Verification items for the finished model (mm, model axes). Face numbers are marked on the shaded views. A direction names the side the tool comes from. Give positions to 0.01 mm unless a question says otherwise; leave off trailing zeros. Loops run counter-clockwise (first coordinate to the right, second up) from the corner with the lowest first, then second, coordinate; pieces in that order, holes last. Notation, with made-up numbers: M -14.75,39.25 L 8.25,39.25 A19 cw 8.25,54.25 Z; hole C -0.5,73.25 d3. An arc over 180 degrees is marked long. Use CSV: the item, a comma, the result in double quotes.
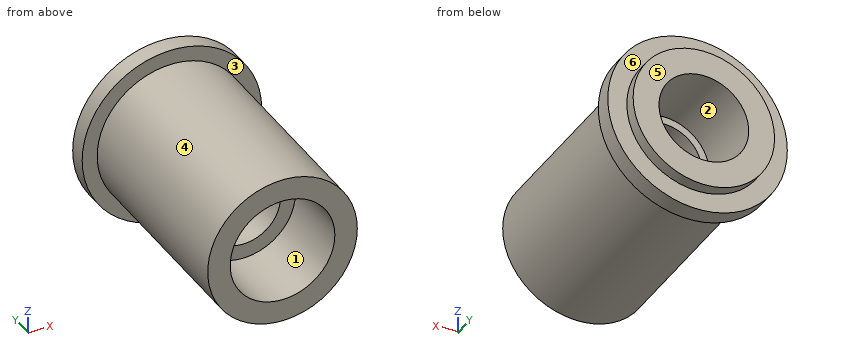
from build123d import *

# Parameters (mm, degrees)
F0_R     = 9.525
F0_R_2   = 7.5057
F0_R_3   = 4.7625
F1_DEPTH = 25.4
F2_R     = 5.55625
F3_DEPTH = 7.9375
F2_R_2   = 9.525
F2_R_3   = 7.9375
F5_DEPTH = 22.225
F6_DEPTH = 1.27
F7_DEPTH = 7.9375
F8_D     = 7.9375


with BuildPart() as f1:
    # F0 (on Front) → F1 (new body)
    with BuildSketch(Plane.XZ):
        Circle(F0_R)
        Circle(F0_R_2, mode=Mode.SUBTRACT)
        Circle(F0_R_2)
        Circle(F0_R_3, mode=Mode.SUBTRACT)
        Circle(F0_R_3)
    extrude(amount=F1_DEPTH)

    # F2 (on face) → F3 (cut)
    with BuildSketch(Plane.XZ.offset(25.4)):
        Circle(F2_R)
    extrude(amount=-F3_DEPTH, mode=Mode.SUBTRACT)

    # F2 (on face) → F5 (cut)
    with BuildSketch(Plane.XZ.offset(25.4)):
        Circle(F2_R_2)
        Circle(F2_R_3, mode=Mode.SUBTRACT)
    extrude(amount=-F5_DEPTH, mode=Mode.SUBTRACT)

    # F0 (on Front) → F6 (cut)
    with BuildSketch(Plane.XZ):
        Circle(F0_R)
        Circle(F0_R_2, mode=Mode.SUBTRACT)
    extrude(amount=F6_DEPTH, mode=Mode.SUBTRACT)

    # F0 (on Front) → F7 (cut)
    with BuildSketch(Plane.XZ):
        Circle(F0_R_3)
    extrude(amount=F7_DEPTH, mode=Mode.SUBTRACT)

    # F8 (through all)
    with Locations(Plane.XZ.offset(17.4625)):
        with Locations((0, 0)):
            Hole(F8_D / 2)


solid = f1.part
(1) Section check B-B on z = 0. Record the cut outline in (x, y) (1 decimal), plus the area to 3 significant figures.
Calculated:
outline,"M -9.5,-3.2 L -7.9,-3.2 L -7.9,-25.4 L -5.6,-25.4 L -5.6,-17.5 L -4,-17.5 L -4,-7.9 L -4.8,-7.9 L -4.8,0 L -7.5,0 L -7.5,-1.3 L -9.5,-1.3 Z; M 4,-17.5 L 5.6,-17.5 L 5.6,-25.4 L 7.9,-25.4 L 7.9,-3.2 L 9.5,-3.2 L 9.5,-1.3 L 7.5,-1.3 L 7.5,0 L 4.8,0 L 4.8,-7.9 L 4,-7.9 Z"
area,"169 mm²"
(2) Mould release check, pull along X, two halves, no side actions. Record for the marked faces 1, 2, 3 and 4: released by +X, released by -X, zero draft, split by the parting line, or undercut.
Calculated:
face 1,"undercut"
face 2,"undercut"
face 3,"zero draft"
face 4,"split by the parting line"
(3) Section check A-A on x = 0. Record the cut outline in (y, z) (1 decimal).
Calculated:
outline,"M -25.4,-7.9 L -3.2,-7.9 L -3.2,-9.5 L -1.3,-9.5 L -1.3,-7.5 L 0,-7.5 L 0,-4.8 L -7.9,-4.8 L -7.9,-4 L -17.5,-4 L -17.5,-5.6 L -25.4,-5.6 Z; M -25.4,5.6 L -17.5,5.6 L -17.5,4 L -7.9,4 L -7.9,4.8 L 0,4.8 L 0,7.5 L -1.3,7.5 L -1.3,9.5 L -3.2,9.5 L -3.2,7.9 L -25.4,7.9 Z"
(4) Tool access check on the marked faces 5 and 6. Record the directions out of +Z, -Z, +X, -X, +Y, -Y that give a thin tool (end or side, any length) a straight path to the whole face; none if there is none.
Calculated:
face 5,"+Z, -Z, +X, -X, +Y"
face 6,"+Y"
(5) Depth check by flat-ended pin: pin 1 Ø8 at (y, z) = (-22, -1.5) entering from +X; pin 2 Ø4 at (y, z) = (-5, 5.5) entering from +X; pin 3 Ø1 at (x, z) = (4, 0) entering from +Y. Enter the tip coordinate at first touch or a pass-through.
Calculated:
pin 1,"stops at x = 7.94"
pin 2,"stops at x = 8.29"
pin 3,"stops at y = -7.94"
(6) Section check C-C on z = 6. Record the cut outline in (x, y) (1 decimal), plus the area to 3 significant figures.
Calculated:
outline,"M -7.4,-3.2 L -5.2,-3.2 L -5.2,-25.4 L 5.2,-25.4 L 5.2,-3.2 L 7.4,-3.2 L 7.4,-1.3 L 4.5,-1.3 L 4.5,0 L -4.5,0 L -4.5,-1.3 L -7.4,-1.3 Z"
area,"271 mm²"
(7) Scan lines: L1, parallel to Z at x = 0, y = -22; L2, parallel to Z at x = 0, y = -2 (1 decimal); L3, parallel to X at y = -10.5, z = -0.25. Record each from-to range of solid material in increasing order. Write a range as from..to.
Calculated:
L1,"z = -7.94..-5.56, 5.56..7.94"
L2,"z = -9.5..-4.8, 4.8..9.5"
L3,"x = -7.93..-3.96, 3.96..7.93"
(8) Section check D-D on x = -8.25. Record the cut outline in (y, z) (3 decimals).
Calculated:
outline,"M -3.175,-4.761 L -1.27,-4.761 L -1.27,4.761 L -3.175,4.761 Z"
